Here's how the part is built. I have some questions about the finished solid (model axes, mm). Give positions to 0.01 mm unless a question says otherwise; leave off trailing zeros. Loops run counter-clockwise (first coordinate to the right, second up) from the corner with the lowest first, then second, coordinate; pieces in that order, holes last. Notation, with made-up numbers: (25, 53.25) - (75, 53.25) arc R15 ccw to (75, 68.25) - close; hole circle Ø8 at (83.5, 24.25). An arc over 180 degrees is marked (long way). Return JSON: item names as keys, results as strings. Group by question number.
(1) For P1, Ø2, axis at y = -130, z = 1, coming from the +X side; P2, Ø4, axis at y = -128, z = 1.5, coming from the +X side, each with a flat end and sliding along its axis, tell me the tip position at first contact or that it passes through.
(2) I need wall thicknesses on probe 1 along Y at (x, z) = (1, 5.5); probe 2 along X at (y, z) = (-32, 4.25); probe 3 along Y at (x, z) = (14.5, 7). Which ranges of each line are inside material? Lowest first, please. Write a range as [from, to].
(3) If we section it at B-B (y = 87): Please give me the cut outline in (x, z), then the cut area to 3 significant figures.
(4) If we section it at A-A (x = -53): Please give me the cut outline in (y, z).
Autodesk Inventor part; units mm, degrees
ref_plane "YZ Plane" through (0, 0, 0) normal (1, 0, 0) x (0, 1, 0)
ref_plane "XZ Plane" through (0, 0, 0) normal (0, 1, 0) x (-1, 0, 0)
ref_plane "XY Plane" through (0, 0, 0) normal (0, 0, 1) x (1, 0, 0)
sketch "スケッチ1" plane through (0, 0, 0) normal (0, 0, 1) x (1, 0, 0)
  line L0 (-231, 185) -> (231, 185)
  line L1 (231, 185) -> (231, -185)
  line L2 (231, -185) -> (-231, -185)
  line L3 (-231, -185) -> (-231, 185)
  line L4 (-231, 185) -> (231, -185) construction
  line L5 (231, 185) -> (-231, -185) construction
  point P0 (0, 0)
  dimension "d0" = 462
  dimension "d1" = 370
extrude "押し出し1" add sketch "スケッチ1" along normal blind 8.35
sketch "スケッチ2" plane through (0, 0, 8.35) normal (0, 0, 1) x (1, 0, 0)
  line L0 (-200, 155) -> (200, 155)
  line L1 (200, 155) -> (200, -155)
  line L2 (200, -155) -> (-200, -155)
  line L3 (-200, -155) -> (-200, 155)
  line L4 (-200, 155) -> (200, -155) construction
  line L5 (200, 155) -> (-200, -155) construction
  point P0 (0, 0)
  dimension "d4" = 400
  dimension "d5" = 310
extrude "押し出し2" cut sketch "スケッチ2" against normal blind 8.35
fillet "フィレット1" radius 3 11 edges at (0, 185, 8.35) (231, 185, 4.175) (0, 185, 0) (-231, 185, 4.175) (-231, 0, 8.35) (231, 0, 8.35) (231, 0, 0) (231, -185, 4.175) (0, -185, 8.35) (-231, -185, 4.175) (-231, 0, 0)
properties part number "upperGom"
Values:
{
 "1": {"P1": "x = 230.83", "P2": "x = 231"},
 "2": {"probe 1": "[-185, -155], [155, 185]", "probe 2": "[-231, -200], [200, 231]", "probe 3": "[-184.51, -155], [155, 184.51]"},
 "3": {"outline": "(-231, 3) arc R3 ccw to (-228, 0) - (-200, 0) - (-200, 8.35) - (-228, 8.35) arc R3 ccw to (-231, 5.35) - close; (200, 0) - (228, 0) arc R3 ccw to (231, 3) - (231, 5.35) arc R3 ccw to (228, 8.35) - (200, 8.35) - close", "area": "510 mm2"},
 "4": {"outline": "(-185, 0) - (-155, 0) - (-155, 8.35) - (-182, 8.35) arc R3 ccw to (-185, 5.35) - close; (155, 0) - (182, 0) arc R3 ccw to (185, 3) - (185, 5.35) arc R3 ccw to (182, 8.35) - (155, 8.35) - close"}
}
